Read the model definition and answer for the solid it produces. Units are mm, in the model's axes. Give positions to 0.01 mm unless a question says otherwise; leave off trailing zeros. Write each loop counter-clockwise with the first axis right and the second up, starting at its lowest first coordinate (ties: lowest second). Pieces come first, ordered by that corner, then holes. Notation, with made-up numbers: (42.5, 70.5) -> (46.5, 70.5) arc R19 cw to (46.5, 86.5) -> close; hole circle Ø6 at (12.25, 7.5). An arc over 180 degrees is marked (long way). Write item = value, one per line.
Autodesk Inventor part; units mm, degrees
ref_plane "YZ Plane" through (0, 0, 0) normal (1, 0, 0) x (0, 1, 0)
ref_plane "XZ Plane" through (0, 0, 0) normal (0, 1, 0) x (-1, 0, 0)
ref_plane "XY Plane" through (0, 0, 0) normal (0, 0, 1) x (1, 0, 0)
sketch "Sketch1" plane through (0, 0, 0) normal (1, 0, 0) x (0, 1, 0)
  line L0 (0, -19.05) -> (0, -190.5)
  line L1 (12.7, -203.2) -> (27.1441, -203.2)
  line L2 (63.5, -203.2) -> (63.5, -19.05) construction
  line L3 (0, -25.4) -> (19.05, -25.4) construction
  line L4 (19.05, -25.4) -> (19.05, -63.5) construction
  line L5 (19.05, -63.5) -> (19.05, -101.6) construction
  line L6 (19.05, -101.6) -> (19.05, -139.7) construction
  line L7 (19.05, -25.4) -> (31.75, -25.4) construction
  line L8 (31.75, -25.4) -> (44.45, -25.4) construction
  line L9 (44.45, -25.4) -> (44.45, -63.5) construction
  line L10 (44.45, -63.5) -> (44.45, -101.6) construction
  line L11 (44.45, -101.6) -> (44.45, -139.7) construction
  line L12 (31.75, -25.4) -> (31.75, -63.5) construction
  line L13 (31.75, -63.5) -> (31.75, -101.6) construction
  line L14 (31.75, -101.6) -> (31.75, -139.7) construction
  line L15 (31.75, -139.7) -> (31.75, -161.925) construction
  line L16 (44.45, 0) -> (19.05, 0)
  arc A0 (19.05, 0) -> (0, -19.05) centre (19.05, -19.05) ccw
  arc A1 (63.5, -19.05) -> (44.45, 0) centre (44.45, -19.05) ccw
  line L17 (31.75, -161.925) -> (67.5523, -148.894) construction
  line L18 (31.75, -161.925) -> (69.85, -161.925) construction
  line L19 (19.05, -139.7) -> (19.05, -177.8) construction
  line L20 (31.75, -161.925) -> (19.8159, -166.2687) construction
  line L21 (31.75, -161.925) -> (44.45, -161.925) construction
  line L22 (19.8159, -166.2687) -> (15.4722, -154.3346) construction
  line L23 (15.4722, -154.3346) -> (3.5382, -158.6782) construction
  line L24 (3.5382, -158.6782) -> (2.93, -157.0074)
  line L25 (44.45, -101.6) -> (44.45, -120.65)
  line L26 (44.45, -120.65) -> (63.5, -120.65)
  line L27 (63.5, -120.65) -> (63.5, -133.35)
  line L28 (63.5, -133.35) -> (61.722, -133.35)
  line L29 (63.5, -19.05) -> (63.5, -95.25)
  line L30 (63.5, -203.2) -> (82.55, -203.2)
  line L31 (82.55, -203.2) -> (82.55, -184.15)
  line L32 (63.5, -95.25) -> (63.5, -117.475)
  line L33 (63.5, -117.475) -> (82.55, -117.475) construction
  arc A2 (82.55, -117.475) -> (63.5, -95.25) centre (61.8713, -115.9228) ccw
  line L34 (82.55, -117.475) -> (82.55, -179.7494)
  line L35 (82.55, -203.2) -> (31.75, -203.2)
  line L36 (36.0626, -201.5828) -> (78.4296, -185.6951)
  arc A3 (0, -190.5) -> (12.7, -203.2) centre (12.7, -190.5) ccw
  arc A4 (78.4296, -185.6951) -> (82.55, -179.7494) centre (76.2, -179.7494) ccw
  arc A5 (27.1441, -203.2) -> (36.0626, -201.5828) centre (27.1441, -177.8) ccw
  line L37 (31.75, -25.4) -> (31.75, -4.445) construction
  point P0 (0, 0)
  point P1 (0, -203.2)
  point P2 (63.5, 0)
  point P3 (63.5, -134.85)
  point P4 (63.5, -181.028)
  point P5 (63.5, -191.2938)
  dimension "d0" = 203.2
  dimension "d1" = 63.5
  dimension "d13" = 38.1
  dimension "d14" = 38.1
  dimension "d15" = 38.1
  dimension "d17" = 12.7
  dimension "d18" = 12.7
  dimension "d19" = 22.225
  dimension "d28" = 19.05
  dimension "d29" = 19.05
  dimension "d31" = 38.1
  dimension "d32" = 20
  dimension "d33" = 38.1
  dimension "d34" = 38.1
  dimension "d35" = 38.1
  dimension "d36" = 38.1
  dimension "d40" = 12.7
  dimension "d41" = 160
  dimension "d42" = 12.7
  dimension "d43" = 12.7
  dimension "d44" = 1.778
  dimension "d45" = 19.05
  dimension "d46" = 19.05
  dimension "d48" = 12.7
  dimension "d49" = 1.778
  dimension "d50" = 76.2
  dimension "d51" = 19.05
  dimension "d52" = 19.05
  dimension "d53" = 22.225
  dimension "d54" = 50.8
  dimension "d55" = 12.7
  dimension "d56" = 6.35
  dimension "d57" = 25.4
  dimension "d58" = 20.955
extrude "Extrusion1" add sketch "Sketch1" along normal blind 1.5875
hole "Hole2" at (0, 19.05, -25.4) at (0, 19.05, -63.5) at (0, 19.05, -101.6) at (0, 19.05, -139.7) at (0, 44.45, -25.4) at (0, 31.75, -25.4) at (0, 31.75, -63.5) at (0, 44.45, -63.5) at (0, 31.75, -101.6) at (0, 44.45, -101.6) at (0, 31.75, -139.7) at (0, 44.45, -139.7) at (0, 31.75, -161.925) at (0, 67.5523, -148.894) at (0, 19.05, -177.8) at (0, 15.4722, -154.3346) at (0, 2.93, -157.0074) at (0, 63.5, -120.65) at (0, 61.722, -133.35) at (0, 31.75, -4.445) direction (1, 0, 0) diameter 4.7625 end through all
properties part number "dtplate"
(1) The part is cut by section A-A on z = -120.65. Determine the outline of the cut face in (x, y).
Checks:
outline = (0, 0) -> (1.59, 0) -> (1.59, 61.12) -> (0, 61.12) -> close; (0, 65.88) -> (1.59, 65.88) -> (1.59, 82.55) -> (0, 82.55) -> close
(2) For a pull along Z with two mould halves and no side action, classify faces 1 (the flat face through (1.588, 41, -100)), 2 (the flat face through (0.78, 56.95, -193.75)), 3 (the cylindrical face through (0.805, 30.141, -65.255)) as released by +Z, released by -Z, zero draft, split by the parting line, or undercut.
Checks:
face_1 = zero draft
face_2 = released by -Z
face_3 = undercut
(3) The part is cut by section B-B on z = -25.4. Determine the outline of the cut face in (x, y).
Checks:
outline = (0, 0) -> (1.59, 0) -> (1.59, 16.67) -> (0, 16.67) -> close; (0, 21.43) -> (1.59, 21.43) -> (1.59, 29.37) -> (0, 29.37) -> close; (0, 34.13) -> (1.59, 34.13) -> (1.59, 42.07) -> (0, 42.07) -> close; (0, 46.83) -> (1.59, 46.83) -> (1.59, 63.5) -> (0, 63.5) -> close
(4) The part is cut by section C-C on x = 0.4. Count the separate pieces of the cut face and the enclosed holes in it, plus the area to 3 significant figures.
Checks:
separate_pieces = 1
enclosed_holes = 20
area = 13,800 mm²
(5) Consider L1, parallel to Y at x = 1.2, z = -25.4; L2, parallel to Y at x = 0.55, z = -24.5; L3, parallel to Y at x = 0.8, z = -133.35. Determine where each line is inside the solid, lowest interval first.
Checks:
L1 = 0 to 16.67, 21.43 to 29.37, 34.13 to 42.07, 46.83 to 63.5
L2 = 0 to 16.85, 21.25 to 29.55, 33.95 to 42.25, 46.65 to 63.5
L3 = 0 to 59.34, 64.1 to 82.55
(6) The part is cut by section D-D on y = 31.75. Determine the outline of the cut face in (x, z), plus the area to 3 significant figures.
Checks:
outline = (0, -202.78) -> (1.59, -202.78) -> (1.59, -164.31) -> (0, -164.31) -> close; (0, -159.54) -> (1.59, -159.54) -> (1.59, -142.08) -> (0, -142.08) -> close; (0, -137.32) -> (1.59, -137.32) -> (1.59, -103.98) -> (0, -103.98) -> close; (0, -99.22) -> (1.59, -99.22) -> (1.59, -65.88) -> (0, -65.88) -> close; (0, -61.12) -> (1.59, -61.12) -> (1.59, -27.78) -> (0, -27.78) -> close; (0, -23.02) -> (1.59, -23.02) -> (1.59, -6.83) -> (0, -6.83) -> close; (0, -2.06) -> (1.59, -2.06) -> (1.59, 0) -> (0, 0) -> close
area = 277 mm²
(7) Given P1, Ø0.5, axis at x = 0.5, z = -134, coming from the +Y side; P2, Ø0.5, axis at x = 1, z = -68, coming from the +Y side, each flat-ended and moving along its own axis, determine where each tip first touches the part or whether it passes through.
Checks:
P1 = 82.55
P2 = 63.5
